```python
from build123d import *

# Parameters (mm, degrees)
CUT_EXTRUDE1_DEPTH = 0.762
CIRPATTERN1_COUNT  = 6
CUT_SWEEP1_PITCH   = 0.5715


with BuildPart() as part:
    # Sketch1 → Revolve1 (revolve)
    with BuildSketch(Plane.XY, mode=Mode.PRIVATE) as revolve1_sk:
        Polygon((0, 0), (5.715, 0), (5.715, 1.4478), (1.143, 1.4478), (0.4064, 2.667), (0, 2.667), align=None)
    revolve(revolve1_sk.sketch.rotate(Axis((0, 0, 0), (-1, 0, 0)), 90), axis=Axis((0, 0, 0), (-1, 0, 0)))

    # Sketch2 → Cut-Extrude1 (cut)
    with BuildSketch(Plane.ZY):
        Polygon((0, 1.778), (0.513264389, 0.889), (1.539793168, 0.889), (0, 0), align=None)
    cut_extrude1 = extrude(amount=-CUT_EXTRUDE1_DEPTH, mode=Mode.SUBTRACT)

    # CirPattern1: Cut-Extrude1 ×6 about axis
    cirpattern1_axis = Axis((0, 0, 0), (1, 0, 0))
    for i in range(1, CIRPATTERN1_COUNT):
        add(cut_extrude1.rotate(cirpattern1_axis, i * 360 / CIRPATTERN1_COUNT), mode=Mode.SUBTRACT)

    # Cut-Sweep1: arcs per turn and ends read off the stored shape
    # Cut-Sweep1: the profile of Sketch5 profile screwed along a right-hand helix through 8.75 turns, 6 arcs to a turn; built about Z, then put on its axis
    cut_sweep1_z = Axis((0, 0, 0), (0, 0, 1))
    cut_sweep1_corners = [(1.448004946, 5.56e-06, -0.444420005), (1.448004946, 5.56e-06, -0.698580005), (0.971454946, 3.73e-06, -0.571500005)]
    with BuildLine(mode=Mode.PRIVATE) as cut_sweep1_profile:
        Line(cut_sweep1_corners[0], cut_sweep1_corners[1])
        Line(cut_sweep1_corners[1], cut_sweep1_corners[2])
        Line(cut_sweep1_corners[2], cut_sweep1_corners[0])
    cut_sweep1_cap = Face(cut_sweep1_profile.wire())
    cut_sweep1_turn_angles = [0, 30, 60, 90, 120, 150, 180, 210, 240, 270, 300, 330, 360]
    cut_sweep1_turn_weights = [1, 0.8660254037844387, 1, 0.8660254037844387, 1, 0.8660254037844387, 1, 0.8660254037844387, 1, 0.8660254037844387, 1, 0.8660254037844387, 1]
    cut_sweep1_turn_rails = [Edge.make_bspline([Vector(p[0], p[1], 0).rotate(cut_sweep1_z, cut_sweep1_turn_angles[k]) / cut_sweep1_turn_weights[k] + Vector(0, 0, p[2] + CUT_SWEEP1_PITCH * cut_sweep1_turn_angles[k] / 360) for k in range(13)], [0, 0, 0, 1, 1, 2, 2, 3, 3, 4, 4, 5, 5, 6, 6, 6], 2, cut_sweep1_turn_weights) for p in cut_sweep1_corners]
    cut_sweep1_turn_sides = [Face.make_surface_from_curves(cut_sweep1_turn_rails[p[0]], cut_sweep1_turn_rails[p[1]]) for p in [(0, 1), (1, 2), (2, 0)]]
    cut_sweep1_last_angles = [2880, 2910, 2940, 2970, 3000, 3030, 3060, 3090, 3120, 3135, 3150]
    cut_sweep1_last_weights = [1, 0.8660254037844387, 1, 0.8660254037844387, 1, 0.8660254037844387, 1, 0.8660254037844387, 1, 0.9659258262890683, 1]
    cut_sweep1_last_rails = [Edge.make_bspline([Vector(p[0], p[1], 0).rotate(cut_sweep1_z, cut_sweep1_last_angles[k]) / cut_sweep1_last_weights[k] + Vector(0, 0, p[2] + CUT_SWEEP1_PITCH * cut_sweep1_last_angles[k] / 360) for k in range(11)], [0, 0, 0, 1, 1, 2, 2, 3, 3, 4, 4, 5, 5, 5], 2, cut_sweep1_last_weights) for p in cut_sweep1_corners]
    cut_sweep1_last_sides = [Face.make_surface_from_curves(cut_sweep1_last_rails[p[0]], cut_sweep1_last_rails[p[1]]) for p in [(0, 1), (1, 2), (2, 0)]]
    cut_sweep1 = Plane(origin=(5.715, 0, 0), x_dir=(0, -0.2079116908177638, 0.9781476007338047), z_dir=(-1, 0, 0)) * Solid(Shell([*[p.moved(Location((0, 0, CUT_SWEEP1_PITCH * i))) for i in range(8) for p in cut_sweep1_turn_sides], *cut_sweep1_last_sides, cut_sweep1_cap, cut_sweep1_cap.rotate(cut_sweep1_z, 3150).moved(Location((0, 0, CUT_SWEEP1_PITCH * 3150 / 360)))]))
    add(cut_sweep1, mode=Mode.SUBTRACT)


solid = part.part
```
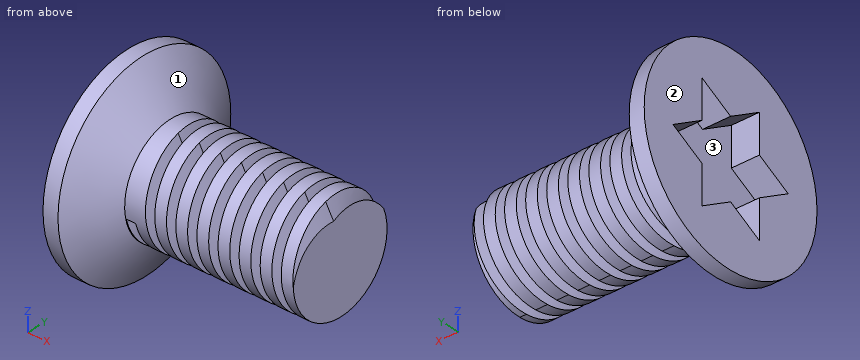
Part model, mm, in its own coordinate system. Face numbers are marked on the shaded views. Coordinates: 2 decimals unless noted, no trailing zeros. Write item = value, one per line. Start each with the question number.
Item 1: Mould opens along Z. For the marked faces 1, 2 and 3 say: released by +Z, released by -Z, zero draft, split by the parting line, or undercut.
Item 2: Wall check: L1, parallel to X at y = 0.6, z = 0.1 (3 decimals); L2, parallel to X at y = 0.5, z = 1.45; L3, parallel to Z at x = 0.3, y = -0.45. Give the ranges that are in metal, low to high. Write a range as from..to.
Item 3: Flat gauge pins, fed straight in: pin 1 Ø0.8 at (x, z) = (0.5, 1) entering from -Y; pin 2 Ø1.5 at (x, z) = (2, -1.5) entering from +Y; pin 3 Ø2 at (x, z) = (1.5, 0.5) entering from +Y. Where does each tip first touch, or does it go through?
The answers:
q1.face_1 = split by the parting line
q1.face_2 = zero draft
q1.face_3 = undercut
q2.L1 = 0.762..5.715
q2.L2 = 0..1.09
q2.L3 = -2.63..-1.29, 1.29..2.63
q3.pin_1 = -2.6
q3.pin_2 = 1.24
q3.pin_3 = 2.47
